Here's how the part is built. I have some questions about the finished solid (model axes, mm). A direction names the side the tool comes from. Round coordinates to 2 decimals unless told otherwise and drop trailing zeros. Loops run counter-clockwise (first coordinate to the right, second up) from the corner with the lowest first, then second, coordinate; pieces in that order, holes last. Notation, with made-up numbers: M -24,31.5 L 33,31.5 A22 cw 33,57.5 Z; hole C 36,-13 d5. An arc over 180 degrees is marked long. Use a Markdown table: item, result.
```python
from build123d import *

# Parameters (mm, degrees)
F2_SIZE  = 0.5
F4_DEPTH = 13.001


with BuildPart() as f1:
    # F0 (on Front) → F1 (revolve)
    with BuildSketch(Plane.XZ):
        Polygon((1.19, 5.79), (1.19, -5), (3, -5), (3, 0), (4.04, 0), (4.04, 4.463661), (0.325, 8), (0.2, 8), (0.2, 7.5), align=None)
    revolve(axis=Axis((0, 0, 0.76721), (0, 0, -1)))

    # F2
    f2_edges = [f1.edges().sort_by_distance(p)[0] for p in [
        (-3, 0, -5),
    ]]
    chamfer(f2_edges, length=F2_SIZE)

    # F3 (on face) → F4 (cut, through all)
    with BuildSketch(Plane.XY.offset(8)):
        Polygon((5.229439, 4.649782), (3.5, 4.649782), (3.5, 4.01771), (5.229439, 3.019218), align=None)
        Polygon((3.5, 2.020726), (3.5, 4.01771), (1.729439, 5.039944), (0, 4.041452), align=None)
        Polygon((6.746156, 2.143541), (5.229439, 3.019218), (5.229439, 1.022234), (5.881436, 0.645803), align=None)
        Polygon((5.229439, 1.022234), (3.5, 2.020726), (3.5, -2.020726), (5.229439, -1.022234), align=None)
        Polygon((0, 6.038436), (1.729439, 5.039944), (2.381436, 5.416375), (1.516717, 6.914113), align=None)
        Polygon((3.5, -4.01771), (3.5, -2.020726), (0, -4.041452), (1.729439, -5.039944), align=None)
        Polygon((-3.5, 2.020726), (0, 4.041452), (-1.729439, 5.039944), (-3.5, 4.01771), align=None)
        Polygon((-1.729439, 5.039944), (0, 6.038436), (-1.41211, 6.853717), (-2.276829, 5.35598), align=None)
        Polygon((5.776829, -0.706198), (5.229439, -1.022234), (5.229439, -3.019218), (6.641548, -2.203936), align=None)
        Polygon((5.229439, -3.019218), (3.5, -4.01771), (3.5, -4.770572), (5.229439, -4.770572), align=None)
        Polygon((-1.729439, -5.039944), (0, -4.041452), (-3.5, -2.020726), (-3.5, -4.01771), align=None)
        Polygon((-3.5, -2.020726), (-3.5, 2.020726), (-5.229439, 1.022234), (-5.229439, -1.022234), align=None)
        Polygon((2.276829, -5.35598), (1.729439, -5.039944), (0, -6.038436), (1.41211, -6.853717), align=None)
        Polygon((0, -6.038436), (-1.729439, -5.039944), (-2.381436, -5.416375), (-1.516717, -6.914113), align=None)
        Polygon((-5.229439, 3.019218), (-3.5, 4.01771), (-3.5, 4.770572), (-5.229439, 4.770572), align=None)
        Polygon((-5.776829, 0.706198), (-5.229439, 1.022234), (-5.229439, 3.019218), (-6.641548, 2.203936), align=None)
        Polygon((-3.5, -4.649782), (-3.5, -4.01771), (-5.229439, -3.019218), (-5.229439, -4.649782), align=None)
        Polygon((-5.229439, -3.019218), (-5.229439, -1.022234), (-5.881436, -0.645803), (-6.746156, -2.143541), align=None)
    extrude(amount=-F4_DEPTH, mode=Mode.SUBTRACT)


solid = f1.part
```
Q1. I need wall thicknesses on line 1 (X direction, y = 0, z = 2.5); line 2 (X direction, y = 0, z = -2.75). Which ranges of each line are inside material? Lowest first, please. Write a range as from..to.
Return value:
| item | result |
|---|---|
| line 1 | x = -3.5..-1.19, 1.19..3.5 |
| line 2 | x = -3..-1.19, 1.19..3 |
Q2. Imagine slicing it at A-A, the plane y = 0. Please give me the cut outline in (x, z) (3 decimals).
Return value:
| item | result |
|---|---|
| outline | M -3.5,0 L -3,0 L -3,-4.5 L -2.5,-5 L -1.19,-5 L -1.19,5.79 L -0.2,7.5 L -0.2,8 L -0.325,8 L -3.5,4.978 Z; M 0.2,7.5 L 1.19,5.79 L 1.19,-5 L 2.5,-5 L 3,-4.5 L 3,0 L 3.5,0 L 3.5,4.978 L 0.325,8 L 0.2,8 Z |
Q3. Will these pins go through, and if not, where does the flat tip stop? P1, Ø4, axis at x = -2.5, z = -2.5, coming from the -Y side; P2, Ø2, axis at x = 1.5, y = -2.5, coming from the +Z side.
Return value:
| item | result |
|---|---|
| P1 | stops at y = -2.96 |
| P2 | stops at z = 6.49 |
Q4. We'd pull the mould along Y, two halves only. Please class faces 3 (the cylindrical face through (-3, 0, -2)), 4 (the conical face through (-0.104, 0.47, 7.013)), 5 (the flat face through (-1.8, 3, 2.5)), 6 (the flat face through (3.5, 0, 3)): pulls with the +Y half, pulls with the -Y half, needs draft (parallel to the pull), parting line crosses it, or undercut.
Return value:
| item | result |
|---|---|
| face 3 | parting line crosses it |
| face 4 | undercut |
| face 5 | pulls with the +Y half |
| face 6 | needs draft |
Q5. For faces 1 (the flat face through (1, 3, 0)), 2 (the flat face through (1.8, -3, 2.5)), which set-ups out of +Z, -Z, +X, -X, +Y, -Y let a thin tool reach every point of the face, with its end or its side?
Return value:
| item | result |
|---|---|
| face 1 | -Z |
| face 2 | +Z, -Z, +X, -Y |
